Here's the drawing with two shaded views (mm, measured from the low corner). I have some questions. A direction names the side the tool comes from. Give positions to 0.01 mm unless a question says otherwise; leave off trailing zeros. Loops run counter-clockwise (first coordinate to the right, second up) from the corner with the lowest first, then second, coordinate; pieces in that order, holes last. Notation, with made-up numbers: M 80,-34 L 108,-34 A33 ccw 108,-6 Z; hole C -27.5,79 d2. An arc over 180 degrees is marked long. Use a Markdown table: item, result. Add a question column.
1) Which directions (+Z, -Z, +X, -X, +Y, -Y) give clear straight access to the entire face, cutting with the end or side of a thin tool? Please do the marked faces 1 and 2.
2) Suppose I cut it at A-A on x = 17. List the corners of the cut face in (y, z) for me.
3) We'd pull the mould along Y, two halves only. Please class the marked faces 3, 4 and 5: +Y half, -Y half, draft (parallel to the pull), parting line (faces both ways), or undercut.
4) Will these pins go through, and if not, where does the flat tip stop? pin 1 Ø2 at (x, z) = (26, 9.5) entering from +Y; pin 2 Ø0.8 at (y, z) = (29.5, 7) entering from +X.
5) Suppose I cut it at C-C on y = 4.5. List the corners of the cut face in (x, z) for me, and give its area (3 significant figures).
6) If I drill on line 1 along Y through (x, z) = (17, 7.5); line 2 along Y through (x, z) = (29.5, 3), over which ranges is the centre line in solid material (lowest first)? Write a range as [from, to].
7) Suppose I cut it at D-D on x = 43. List the corners of the cut face in (y, z) for me.
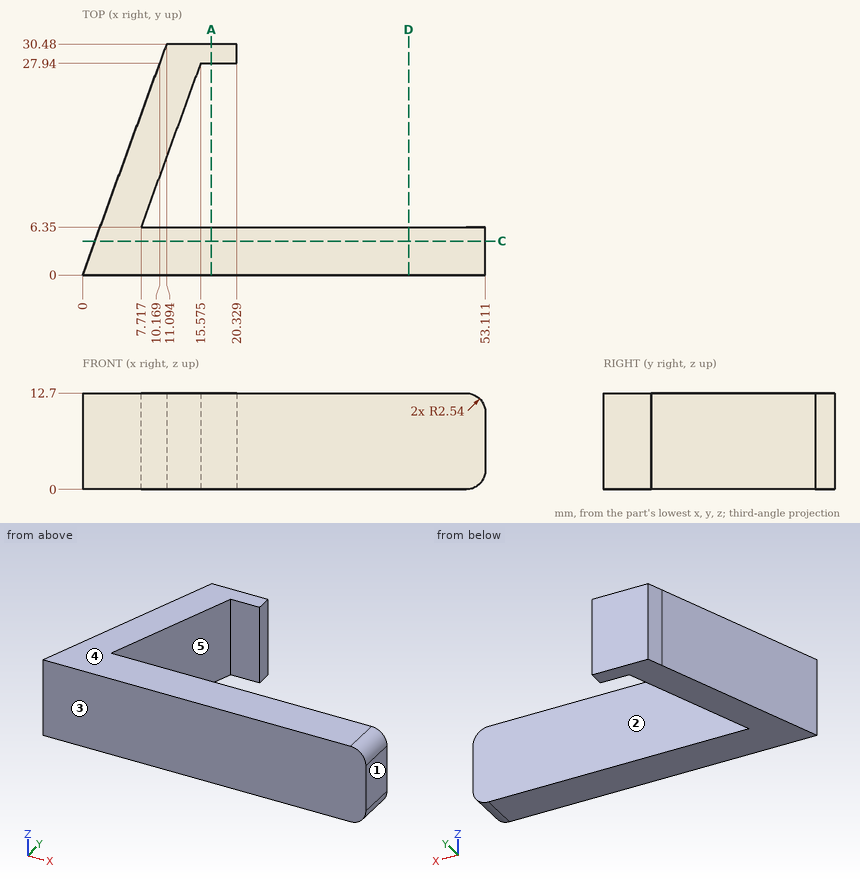
Answer block:
| question | item | result |
|---|---|---|
| 1 | face 1 | +Z, -Z, +X, +Y, -Y |
| 1 | face 2 | +Z, -Z, +X |
| 2 | outline | M 0,0 L 6.35,0 L 6.35,12.7 L 0,12.7 Z; M 27.94,0 L 30.48,0 L 30.48,12.7 L 27.94,12.7 Z |
| 3 | face 3 | -Y half |
| 3 | face 4 | draft |
| 3 | face 5 | undercut |
| 4 | pin 1 | stops at y = 6.35 |
| 4 | pin 2 | stops at x = 20.33 |
| 5 | outline | M 1.64,0 L 50.57,0 A2.54 ccw 53.11,2.54 L 53.11,10.16 A2.54 ccw 50.57,12.7 L 1.64,12.7 Z |
| 5 | area | 651 mm^2 |
| 6 | line 1 | y = [0, 6.35], [27.94, 30.48] |
| 6 | line 2 | y = [0, 6.35] |
| 7 | outline | M 0,0 L 6.35,0 L 6.35,12.7 L 0,12.7 Z |
